Print and shaded views of the part. All mm, measured from the part's lowest x, y and z. A direction names the side the tool comes from. Round coordinates to 2 decimals unless told otherwise and drop trailing zeros. Loops run counter-clockwise (first coordinate to the right, second up) from the corner with the lowest first, then second, coordinate; pieces in that order, holes last. Notation, with made-up numbers: (58.25, 2) -> (117.25, 2) arc R24 ccw to (117.25, 27) -> close; hole circle Ø1 at (76.25, -32.5). An arc over 180 degrees is marked (long way). Use a Markdown table: item, result.
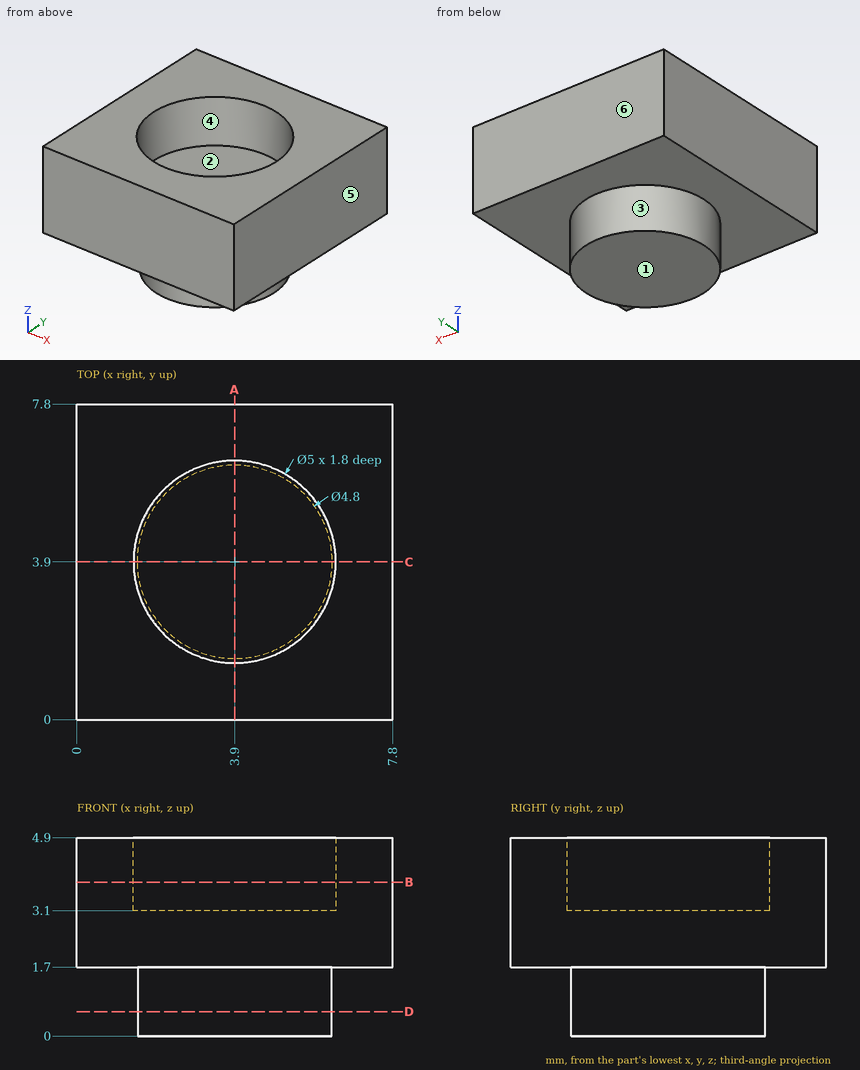
Q1. Drill centre lines: L1, parallel to Y at x = 3.9, z = 3.9; L2, parallel to Z at x = 7, y = 6.75; L3, parallel to Z at x = 3, y = 2.25. Where is each one in solid material? Low to high. Write a range as from..to.
Results list:
| item | result |
|---|---|
| L1 | y = 0..1.4, 6.4..7.8 |
| L2 | z = 1.7..4.9 |
| L3 | z = 0..3.1 |
Q2. Band-saw the part on B-B, the plane z = 3.8. Give the cut face in (x, y).
Results list:
| item | result |
|---|---|
| outline | (0, 0) -> (7.8, 0) -> (7.8, 7.8) -> (0, 7.8) -> close; hole circle Ø5 at (3.9, 3.9) |
Q3. Band-saw the part on A-A, the plane x = 3.9. Give the cut face in (y, z).
Results list:
| item | result |
|---|---|
| outline | (0, 1.7) -> (1.5, 1.7) -> (1.5, 0) -> (6.3, 0) -> (6.3, 1.7) -> (7.8, 1.7) -> (7.8, 4.9) -> (6.4, 4.9) -> (6.4, 3.1) -> (1.4, 3.1) -> (1.4, 4.9) -> (0, 4.9) -> close |
Q4. Band-saw the part on D-D, the plane z = 0.6. Give the cut face in (x, y).
Results list:
| item | result |
|---|---|
| outline | circle Ø4.8 at (3.9, 3.9) |
Q5. Tool access for the marked faces 1, 2 and 3: list every direction of +Z, -Z, +X, -X, +Y, -Y with a clear straight run to the whole face (end or side of a thin tool).
Results list:
| item | result |
|---|---|
| face 1 | -Z, +X, -X, +Y, -Y |
| face 2 | +Z |
| face 3 | -Z |
Q6. Pull direction X, two halves, no side cores. Call the marked faces 4, 5 and 6: released by +X, released by -X, zero draft, split by the parting line, or undercut.
Results list:
| item | result |
|---|---|
| face 4 | undercut |
| face 5 | released by +X |
| face 6 | zero draft |
